from build123d import *

# Parameters (mm, degrees)
SKETCH1_R           = 108
SKETCH1_R_2         = 22.5
BOSS_EXTRUDE2_DEPTH = 32


with BuildPart() as part:
    # Sketch1 → Boss-Extrude2 (new body)
    with BuildSketch(Plane.XY):
        Circle(SKETCH1_R)
        with BuildLine():
            ThreePointArc((-39.668209022, 13.799753366), (-28.005440993, -32.874640461), (-9.031806484, -77.084598511))
            ThreePointArc((-9.031806484, -77.084598511), (2.596198221, -85.966451462), (16.102221796, -91.595406289))
            ThreePointArc((16.102221796, -91.595406289), (-1.272703942, -92.991291123), (-18.602920008, -91.120422339))
            ThreePointArc((-18.602920008, -91.120422339), (-48.283083898, -79.484236232), (-72.289675848, -58.508142731))
            ThreePointArc((-72.289675848, -58.508142731), (-77.621570163, -12.590195167), (-39.668209022, 13.799753366))
        make_face(mode=Mode.SUBTRACT)
        with BuildLine():
            ThreePointArc((-13.799753366, -39.668209022), (32.874640461, -28.005440993), (77.084598511, -9.031806484))
            ThreePointArc((77.084598511, -9.031806484), (85.966451462, 2.596198221), (91.595406289, 16.102221796))
            ThreePointArc((91.595406289, 16.102221796), (92.991291123, -1.272703942), (91.120422339, -18.602920008))
            ThreePointArc((91.120422339, -18.602920008), (79.484236232, -48.283083898), (58.508142731, -72.289675848))
            ThreePointArc((58.508142731, -72.289675848), (12.590195167, -77.621570163), (-13.799753366, -39.668209022))
        make_face(mode=Mode.SUBTRACT)
        with BuildLine():
            ThreePointArc((13.799753366, 39.668209022), (-32.874640461, 28.005440993), (-77.084598511, 9.031806484))
            ThreePointArc((-77.084598511, 9.031806484), (-85.966451462, -2.596198221), (-91.595406289, -16.102221796))
            ThreePointArc((-91.595406289, -16.102221796), (-92.991291123, 1.272703942), (-91.120422339, 18.602920008))
            ThreePointArc((-91.120422339, 18.602920008), (-79.484236232, 48.283083898), (-58.508142731, 72.289675848))
            ThreePointArc((-58.508142731, 72.289675848), (-12.590195167, 77.621570163), (13.799753366, 39.668209022))
        make_face(mode=Mode.SUBTRACT)
        Circle(SKETCH1_R_2, mode=Mode.SUBTRACT)
        with BuildLine():
            ThreePointArc((39.668209022, -13.799753366), (28.005440993, 32.874640461), (9.031806484, 77.084598511))
            ThreePointArc((9.031806484, 77.084598511), (-2.596198221, 85.966451462), (-16.102221796, 91.595406289))
            ThreePointArc((-16.102221796, 91.595406289), (1.272703942, 92.991291123), (18.602920008, 91.120422339))
            ThreePointArc((18.602920008, 91.120422339), (48.283083898, 79.484236232), (72.289675848, 58.508142731))
            ThreePointArc((72.289675848, 58.508142731), (77.621570163, 12.590195167), (39.668209022, -13.799753366))
        make_face(mode=Mode.SUBTRACT)
    extrude(amount=BOSS_EXTRUDE2_DEPTH)


solid = part.part
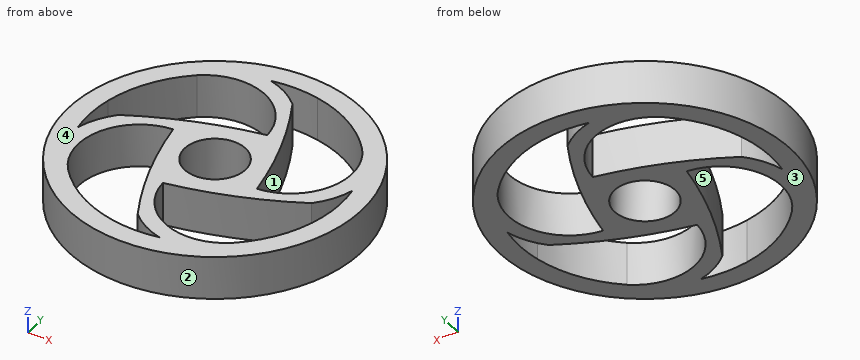
Geometry check sheet. Reference: the model listing, model coordinates, mm. Face numbers are marked on the shaded views. A direction names the side the tool comes from. Round coordinates to 2 decimals unless told otherwise and drop trailing zeros. Loops run counter-clockwise (first coordinate to the right, second up) from the corner with the lowest first, then second, coordinate; pieces in that order, holes last.
Item 1: Gauge pin test, flat ends, axial feed: pin 1 (1 mm diameter, centred on y = -28, z = 27.5, fed in from +X); pin 2 (5 mm diameter, centred on x = -32, z = 11, fed in from -Y); pin 3 (3 mm diameter, centred on y = 84, z = 12, fed in from -X). Record the tip position at first contact, or that the pin passes through.
Item 2: Access from +Z, -Z, +X, -X, +Y, -Y to the whole of each face (thin tool, end or side, straight path). Record for the marked faces 4 and 5.
Item 3: Cross-section at D-D on x = -49. Record the boundary of the cut face in (y, z), then the cut area to 3 significant figures.
Item 4: Thickness scan on line 1 (X direction, y = 65.5, z = 3.5); line 2 (Y direction, x = 0, z = 20); line 3 (X direction, y = -51, z = 15.5). Record the ranges inside material, lowest first.
Item 5: Cross-section at C-C on y = 0. Record the boundary of the cut face in (x, z).
Item 6: Cross-section at B-B on z = 20.5. Record the boundary of the cut face in (x, y).
Item 7: Mould release check, pull along X, two halves, no side actions. Record for the marked faces 1, 2 and 3: pulls with the +X half, pulls with the -X half, needs draft (parallel to the pull), parting line crosses it, or undercut.
Item 8: Cross-section at A-A on x = -88. Record the boundary of the cut face in (y, z).
Answer sheet:
1. pin 1: stops at x = 104.44
1. pin 2: stops at y = -103.89
1. pin 3: stops at x = -69.7
2. face 4: +Z, +X, -X, +Y, -Y
2. face 5: +Z, -Z
3. outline: (-96.24, 0) - (-79.04, 0) - (-79.04, 32) - (-96.24, 32) - close; (12.16, 0) - (22.05, 0) - (22.05, 32) - (12.16, 32) - close; (77.89, 0) - (96.24, 0) - (96.24, 32) - (77.89, 32) - close
3. area: 1,450 mm2
4. line 1: x = -85.87 to -66.02, 3.4 to 14.83, 66.02 to 85.87
4. line 2: y = -108 to -93, -84.37 to -69.13, -37.04 to -22.5, 22.5 to 37.04, 69.13 to 84.37, 93 to 108
4. line 3: x = -95.2 to -76.96, -21.24 to -11.54, 77.77 to 95.2
5. outline: (-108, 0) - (-93, 0) - (-93, 32) - (-108, 32) - close; (-84.37, 0) - (-69.13, 0) - (-69.13, 32) - (-84.37, 32) - close; (-37.04, 0) - (-22.5, 0) - (-22.5, 32) - (-37.04, 32) - close; (22.5, 0) - (37.04, 0) - (37.04, 32) - (22.5, 32) - close; (69.13, 0) - (84.37, 0) - (84.37, 32) - (69.13, 32) - close; (93, 0) - (108, 0) - (108, 32) - (93, 32) - close
6. outline: circle Ø216 at (0, 0); hole (-91.6, -16.1) arc R57 cw to (-77.08, 9.03) arc R300 cw to (13.8, 39.67) arc R45 ccw to (-58.51, 72.29) arc R93 ccw to start; hole (-72.29, -58.51) arc R93 ccw to (16.1, -91.6) arc R57 cw to (-9.03, -77.08) arc R300 cw to (-39.67, 13.8) arc R45 ccw to start; hole circle Ø45 at (0, 0); hole (-16.1, 91.6) arc R57 cw to (9.03, 77.08) arc R300 cw to (39.67, -13.8) arc R45 ccw to (72.29, 58.51) arc R93 ccw to start; hole (-13.8, -39.67) arc R45 ccw to (58.51, -72.29) arc R93 ccw to (91.6, 16.1) arc R57 cw to (77.08, -9.03) arc R300 cw to start
7. face 1: undercut
7. face 2: parting line crosses it
7. face 3: needs draft
8. outline: (-62.61, 0) - (-6.45, 0) - (-6.45, 32) - (-62.61, 32) - close; (30.08, 0) - (62.61, 0) - (62.61, 32) - (30.08, 32) - close
